Could you check a few things on this model? Use its own coordinates, in mm. A direction names the side the tool comes from. Round coordinates to 2 decimals unless told otherwise and drop trailing zeros. Loops run counter-clockwise (first coordinate to the right, second up) from the corner with the lowest first, then second, coordinate; pieces in that order, holes last. Notation, with made-up numbers: M 24.25,74.5 L 35.25,74.5 A23 cw 35.25,109.5 Z; hole C 64,39.5 d5. An arc over 180 degrees is marked long. Return JSON: item names as keys, results as strings. Group by question number.
```python
from build123d import *

# Parameters (mm, degrees)
BOSS_EXTRUDE1_DEPTH = 3
BOSS_EXTRUDE2_DEPTH = 2
BOSS_EXTRUDE3_DEPTH = 17.5
SKETCH4_W           = 8.5
SKETCH4_H           = 3.5
CUT_EXTRUDE1_DEPTH  = 74.816072098


with BuildPart() as part:
    # Sketch1 → Boss-Extrude1 (new body)
    with BuildSketch(Plane.XY):
        with BuildLine():
            Line((0, 0), (46.5, 0))
            Line((46.5, 0), (46.5, 34))
            ThreePointArc((46.5, 34), (23.25, 57.25), (0, 34))
            Line((0, 34), (0, 0))
        make_face()
        with BuildLine():
            Line((2, 2), (2, 34))
            ThreePointArc((2, 34), (23.25, 55.25), (44.5, 34))
            Line((44.5, 34), (44.5, 2))
            Line((44.5, 2), (2, 2))
        make_face(mode=Mode.SUBTRACT)
    extrude(amount=BOSS_EXTRUDE1_DEPTH)

    # Sketch2 → Boss-Extrude2 (add)
    with BuildSketch(Plane.XY.offset(3)):
        with BuildLine():
            Line((0, 34), (0, 0))
            Line((0, 0), (46.5, 0))
            Line((46.5, 0), (46.5, 34))
            ThreePointArc((46.5, 34), (23.25, 57.25), (0, 34))
        make_face()
    extrude(amount=BOSS_EXTRUDE2_DEPTH)

    # Sketch3 → Boss-Extrude3 (add)
    with BuildSketch(Plane(origin=(0, 11.2, 0), x_dir=(1, 0, 0), z_dir=(0, 1, 0))):
        Polygon((2, -2), (3.732050808, -1), (2, 0), align=None)
    boss_extrude3 = extrude(amount=BOSS_EXTRUDE3_DEPTH)

    # Mirror1: Boss-Extrude3 across plane
    add(boss_extrude3.mirror(Plane.ZY.offset(-23.25)))

    # Sketch4 → Cut-Extrude1 (cut, through all)
    with BuildSketch(Plane(origin=(0, 0, 3), x_dir=(-1, 0, 0), z_dir=(0, 0, -1))):
        with Locations((-23.25, 13.75)):
            Rectangle(SKETCH4_W, SKETCH4_H)
    extrude(amount=-CUT_EXTRUDE1_DEPTH, mode=Mode.SUBTRACT)


solid = part.part
```
1. I need wall thicknesses on probe 1 along X at (y, z) = (16, 2.95); probe 2 along Z at (x, y) = (27, 19); probe 3 along Y at (x, z) = (37.5, 2.5). Which ranges of each line are inside material? Lowest first, please.
2. I'm going to push flat-ended pins straight in: pin 1 Ø2 at (x, y) = (19.5, 40.5) entering from -Z; pin 2 Ø1.4 at (x, z) = (3, 0.5) entering from -Y; pin 3 Ø3 at (x, z) = (14.5, 2.5) entering from +Y; pin 4 Ø1.4 at (x, z) = (44, 1) entering from +Y. Where does each tip first touch, or does it pass through?
3. If we section it at C-C, the plane x = 7: Please give me the cut outline in (y, z).
4. If we section it at A-A, the plane x = 23.25: Please give me the cut outline in (y, z), then the cut area to 4 significant figures.
5. We'd pull the mould along X, two halves only. Please class faces 5 (the face through (0, 17, 2)), 6 (the face through (23.761, 57.244, 2.465)), 7 (the face through (23, 0, 2)), 8 (the face through (44, 28.7, 1)): +X half, -X half, draft (parallel to the pull), parting line (faces both ways), or undercut.
6. If we section it at B-B, the plane y = 4: Please give me the cut outline in (x, z), then the cut area to 3 significant figures.
7. On a 3-axis mill with a long thin cutter (end or side, diameter ignored), from which of +Z, -Z, +X, -X, +Y, -Y can I reach the whole of each face in a straight line? I mean faces 1 (the face through (46.5, 17, 2)), 2 (the face through (27.5, 14, 4)), 3 (the face through (3, 28.7, 1)), 4 (the face through (44.5, 18.2, 2.5)). Say none if no direction works.
Geometry results:
{
 "1": {"probe 1": "0 to 2, 44.5 to 46.5", "probe 2": "3 to 5", "probe 3": "0 to 2, 49.76 to 52.37"},
 "2": {"pin 1": "z = 3", "pin 2": "y = 0", "pin 3": "y = 56.09", "pin 4": "y = 45.77"},
 "3": {"outline": "M 0,0 L 2,0 L 2,3 L 47.69,3 L 47.69,0 L 50.63,0 L 50.63,5 L 0,5 Z"},
 "4": {"outline": "M 0,0 L 2,0 L 2,3 L 12,3 L 12,5 L 0,5 Z; M 15.5,3 L 55.25,3 L 55.25,0 L 57.25,0 L 57.25,5 L 15.5,5 Z", "area": "119.5 mm^2"},
 "5": {"face 5": "-X half", "face 6": "parting line", "face 7": "draft", "face 8": "undercut"},
 "6": {"outline": "M 0,0 L 2,0 L 2,3 L 44.5,3 L 44.5,0 L 46.5,0 L 46.5,5 L 0,5 Z", "area": "105 mm^2"},
 "7": {"face 1": "+Z, -Z, +X, +Y, -Y", "face 2": "+Z, -Z", "face 3": "-Z", "face 4": "none"}
}
